Source: CAD feature listing. Evaluate the final solid. Frame: model axes, mm. Face numbers are marked on the shaded views. Coordinates: 2 decimals unless noted, no trailing zeros. Write each loop counter-clockwise with the first axis right and the second up, starting at its lowest first coordinate (ties: lowest second). Pieces come first, ordered by that corner, then holes. Notation, with made-up numbers: M -19,53 L 26,53 A16 cw 26,77 Z; hole C 66.5,-9.75 d6. An arc over 180 degrees is marked long. One line per item, written item: value. Start each with the question number.
Item 1: Cut plane B-B, the plane y = 2.5. Output: boundary loops of the cut face in (x, z).
Item 2: Cut plane A-A, the plane y = 8.5. Output: boundary loops of the cut face in (x, z), then the cut area to 3 significant figures.
Item 3: Pin query (flat end, axial travel): P1, Ø4.5, axis at x = -3, z = 1, coming from the +Y side; P2, Ø1, axis at y = 7.5, z = 7.5, coming from the +X side; P3, Ø1.5, axis at x = -3, z = -1.5, coming from the -Y side. Return the tip coordinate at first contact, or that it passes through.
Item 4: Ray query, L1, parallel to Z at x = 0, y = 8.3; L2, parallel to Z at x = -0.25, y = 4.25; L3, parallel to X at y = 6.5, z = 6. Return the intervals inside material, ascending. Write a range as from..to.
Item 5: Mould query, pull axis Z, two halves, no side actions, for the marked faces 1, 2 and 3. Classes: released by +Z, released by -Z, zero draft, split by the parting line, or undercut.
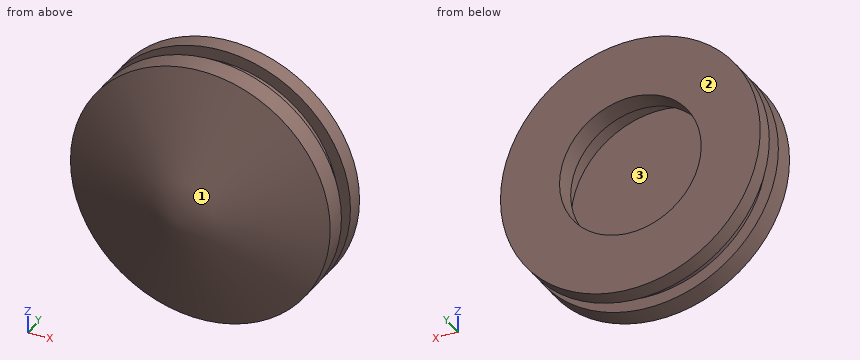
```python
from build123d import *


with BuildPart() as part:
    # Sketch1 → Revolve1 (revolve)
    with BuildSketch(Plane.XY):
        Polygon((0, 0), (0, 8.853672577), (-11, 8.853672577), (-11, 7.353672577), (-10, 7.353672577), (-10, 5.853672577), (-11, 5.853672577), (-11, 4.003672577), align=None)
    revolve(axis=Axis((0, 0, 0), (0, 1, 0)))

    # Sketch2 → Cut-Revolve1 (revolve, cut)
    with BuildSketch(Plane.XY):
        Polygon((0, 4.003672577), (0, 10.003672577), (-6, 10.003672577), (-6, 7.003672577), (-7.5, 7.003672577), (-7.5, 4.003672577), align=None)
    revolve(axis=Axis((0, 4.003672577, 0), (0, 1, 0)), mode=Mode.SUBTRACT)


solid = part.part
```
From the geometry:
1. outline: C 0,0 d13.74
2. outline: C 0,0 d22; hole C 0,0 d12
2. area: 267 mm²
3. P1: stops at y = 4
3. P2: stops at x = 8.49
3. P3: stops at y = 0.95
4. L1: z = -11..-6, 6..11
4. L2: z = -11..-7.5, 7.5..11
4. L3: x = -8..-4.5, 4.5..8
5. face 1: split by the parting line
5. face 2: zero draft
5. face 3: undercut
